Read the model definition and answer for the solid it produces. Units are mm, in the model's axes. A direction names the side the tool comes from. Give positions to 0.01 mm unless a question says otherwise; leave off trailing zeros. Order: outer loops, then holes, each group sorted by start corner. A loop starts at its lowest first (then second) coordinate and runs counter-clockwise, first axis right, second up. Notation, with made-up numbers: (77.25, -3) - (104.25, -3) arc R25 ccw to (104.25, 27) - close; hole circle Ø2 at (-2, -12). An arc over 180 degrees is marked (long way). Write item = value, one per line.
```python
from build123d import *

# Parameters (mm, degrees)
ESQUISSE1_W                  = 101
ESQUISSE1_H                  = 151.5
EXTRUSION1_DEPTH             = 20
CONG_2_R                     = 10.5
CONG_3_R                     = 3.5
COQUE1_T                     = -2
ENL_V_MAT_EXTRU_4_DEPTH      = 21
ENL_V_MAT_EXTRU_1_DEPTH      = 51.5
ENL_V_MAT_EXTRU_1_DEPTH_BACK = 51.5
ENL_V_MAT_EXTRU_2_DEPTH      = 5
ENL_V_MAT_EXTRU_5_DEPTH      = 21


with BuildPart() as part:
    # Esquisse1 → Extrusion1 (new body)
    with BuildSketch(Plane(origin=(0, 0, 0), x_dir=(1, 0, 0), z_dir=(0, 1, 0))):
        Rectangle(ESQUISSE1_W, ESQUISSE1_H)
    extrude(amount=-EXTRUSION1_DEPTH)

    # Congé2
    cong_2_edges = [part.edges().sort_by_distance(p)[0] for p in [
        (0, 0, -75.75),
        (0, 0, 75.75),
    ]]
    fillet(cong_2_edges, radius=CONG_2_R)

    # Congé3
    cong_3_edges = [part.edges().sort_by_distance(p)[0] for p in [
        (-50.5, 0, 0),
        (50.5, 0, 0),
        (-50.5, -3.075378798, 72.674621202),
        (-50.5, -3.075378798, -72.674621202),
        (50.5, -3.075378798, 72.674621202),
        (50.5, -3.075378798, -72.674621202),
        (-50.5, -15.25, -75.75),
        (50.5, -15.25, -75.75),
        (50.5, -15.25, 75.75),
        (-50.5, -15.25, 75.75),
    ]]
    fillet(cong_3_edges, radius=CONG_3_R)

    # Coque1
    coque1_openings = [part.faces().sort_by_distance(p)[0] for p in [
        (0, -20, 0),
    ]]
    offset(amount=COQUE1_T, openings=coque1_openings, kind=Kind.INTERSECTION)

    # Esquisse5 → Enlèv. mat.-Extru.4 (cut, through all)
    with BuildSketch(Plane(origin=(0, 0, 0), x_dir=(-1, 0, 0), z_dir=(0, 1, 0))):
        Polygon((-46.5, -75.75), (-50.5, -75.75), (-50.5, -41.75), (-46.5, -46.75), align=None)
        Polygon((-46.5, 46.75), (-50.5, 41.75), (-50.5, 75.75), (-46.5, 75.75), align=None)
        Polygon((46.5, 75.75), (50.5, 75.75), (50.5, 41.75), (46.5, 46.75), align=None)
        Polygon((46.5, -46.75), (50.5, -41.75), (50.5, -75.75), (46.5, -75.75), align=None)
    extrude(amount=-ENL_V_MAT_EXTRU_4_DEPTH, mode=Mode.SUBTRACT)

    # Esquisse2 → Enlèv. mat.-Extru.1 (cut, two sides)
    with BuildSketch(Plane(origin=(0, 0, 0), x_dir=(0, 0, -1), z_dir=(1, 0, 0))) as enl_v_mat_extru_1_sk:
        with BuildLine():
            Line((-73.75, -10.5), (-73.75, -20))
            Line((-73.75, -20), (73.75, -20))
            Line((73.75, -20), (73.75, -10.5))
            ThreePointArc((73.75, -10.5), (71.26040764, -4.48959236), (65.25, -2))
            Line((65.25, -2), (47.25, -2))
            ThreePointArc((47.25, -2), (39.53637569, -6.929285786), (40.769259302, -16))
            Line((40.769259302, -16), (-40.769259302, -16))
            ThreePointArc((-40.769259302, -16), (-39.53637569, -6.929285786), (-47.25, -2))
            Line((-47.25, -2), (-65.25, -2))
            ThreePointArc((-65.25, -2), (-71.26040764, -4.48959236), (-73.75, -10.5))
        make_face()
    extrude(amount=ENL_V_MAT_EXTRU_1_DEPTH, mode=Mode.SUBTRACT)
    extrude(enl_v_mat_extru_1_sk.sketch, amount=-ENL_V_MAT_EXTRU_1_DEPTH_BACK, mode=Mode.SUBTRACT)

    # Esquisse3 → Enlèv. mat.-Extru.2 (cut)
    with BuildSketch(Plane.ZY.offset(50.5)):
        Polygon((-17.75, -16), (-17.75, -7), (-14.5, 0), (14.5, 0), (17.75, -7), (17.75, -16), align=None)
    extrude(amount=-ENL_V_MAT_EXTRU_2_DEPTH, mode=Mode.SUBTRACT)

    # Esquisse6 → Enlèv. mat.-Extru.5 (cut, through all)
    with BuildSketch(Plane(origin=(0, 0, 0), x_dir=(-1, 0, 0), z_dir=(0, 1, 0))):
        with BuildLine():
            Line((-25.65, 2.65), (-27.85, 2.65))
            ThreePointArc((-27.85, 2.65), (-30.5, 0), (-27.85, -2.65))
            Line((-27.85, -2.65), (-25.65, -2.65))
            ThreePointArc((-25.65, -2.65), (-23, 0), (-25.65, 2.65))
        make_face()
        with BuildLine():
            Line((32.15, -2.65), (34.35, -2.65))
            ThreePointArc((34.35, -2.65), (37, 0), (34.35, 2.65))
            Line((34.35, 2.65), (32.15, 2.65))
            ThreePointArc((32.15, 2.65), (29.5, 0), (32.15, -2.65))
        make_face()
    extrude(amount=-ENL_V_MAT_EXTRU_5_DEPTH, mode=Mode.SUBTRACT)


solid = part.part
```
1. For faces 4 (the face through (-1, -15, 73.75)), 5 (the face through (46.5, -1.8, 65.6)), 6 (the face through (-46.5, -1.8, -65.6)), determine the directions among +Z, -Z, +X, -X, +Y, -Y from which every point of the face is accessible in a straight line to the end or side of a thin tool.
Recorded:
face_4 = +X, -X, -Y
face_5 = +Z, +X, +Y, -Y
face_6 = -Z, -X, +Y, -Y
2. Straight lines are drawn through the part: L1, parallel to Z at x = 15, y = -18.25; L2, parallel to Y at x = 16, z = -52; L3, parallel to X at y = -14, z = -0.5. For each, find the intervals that lie inside material, in ascending order. Write a range as [from, to].
Recorded:
L1 = [-75.75, -73.75], [73.75, 75.75]
L2 = [-2, 0]
L3 = [48.5, 50.5]
3. Section B-B (x = -5) is taken. Determine the outline of the cut face in (y, z), and give its area (3 significant figures).
Recorded:
outline = (-20, -75.75) - (-10.5, -75.75) arc R10.5 ccw to (0, -65.25) - (0, 65.25) arc R10.5 ccw to (-10.5, 75.75) - (-20, 75.75) - (-20, 73.75) - (-10.5, 73.75) arc R8.5 cw to (-2, 65.25) - (-2, -65.25) arc R8.5 cw to (-10.5, -73.75) - (-20, -73.75) - close
area = 359 mm^2
4. Flat-ended cylindrical pins translate along their axes: pin 1 (1.6 mm diameter, centred on y = -1, z = 2.5, fed in from -X); pin 2 (3 mm diameter, centred on x = 36.5, z = -46, fed in from -Y); pin 3 (2 mm diameter, centred on x = 49, z = -20.5, fed in from -Y). Find the tip coordinate at first contact, or state that the pin passes through.
Recorded:
pin_1 = -45.5
pin_2 = -2
pin_3 = -16
5. Determine the mould class of faces 1 (the face through (0.65, -4.56, -71.33)), 2 (the face through (-48.5, -10, 29)), 3 (the face through (-49.474, -9.734, -38.785)) for opening direction Y: +Y half, -Y half, draft (parallel to the pull), parting line (faces both ways), or undercut.
Recorded:
face_1 = -Y half
face_2 = draft
face_3 = undercut
6. Section D-D (z = 23) is taken. Determine the outline of the cut face in (x, y).
Recorded:
outline = (-50.5, -16) - (-48.5, -16) - (-48.5, -3.5) arc R1.5 cw to (-47, -2) - (47, -2) arc R1.5 cw to (48.5, -3.5) - (48.5, -16) - (50.5, -16) - (50.5, -3.5) arc R3.5 ccw to (47, 0) - (-47, 0) arc R3.5 ccw to (-50.5, -3.5) - close
7. Section A-A (z = 0) is taken. Determine the outline of the cut face in (x, y).
Recorded:
outline = (-45.5, -2) - (-37, -2) - (-37, 0) - (-45.5, 0) - close; (-29.5, -2) - (23, -2) - (23, 0) - (-29.5, 0) - close; (30.5, -2) - (47, -2) arc R1.5 cw to (48.5, -3.5) - (48.5, -16) - (50.5, -16) - (50.5, -3.5) arc R3.5 ccw to (47, 0) - (30.5, 0) - close
8. Section C-C (y = -5.5) is taken. Determine the outline of the cut face in (x, z), and give its area (3 significant figures).
Recorded:
outline = (-50.5, -40.38) - (-48.5, -40.38) - (-48.5, -17.05) - (-50.5, -17.05) - close; (-50.5, 17.05) - (-48.5, 17.05) - (-48.5, 40.38) - (-50.5, 40.38) - close; (-46.5, -74.48) - (46.5, -74.48) - (46.5, -72.12) - (-46.5, -72.12) - close; (-46.5, 72.12) - (46.5, 72.12) - (46.5, 74.48) - (-46.5, 74.48) - close; (48.5, -40.38) - (50.5, -40.38) - (50.5, 40.38) - (48.5, 40.38) - close
area = 694 mm^2
